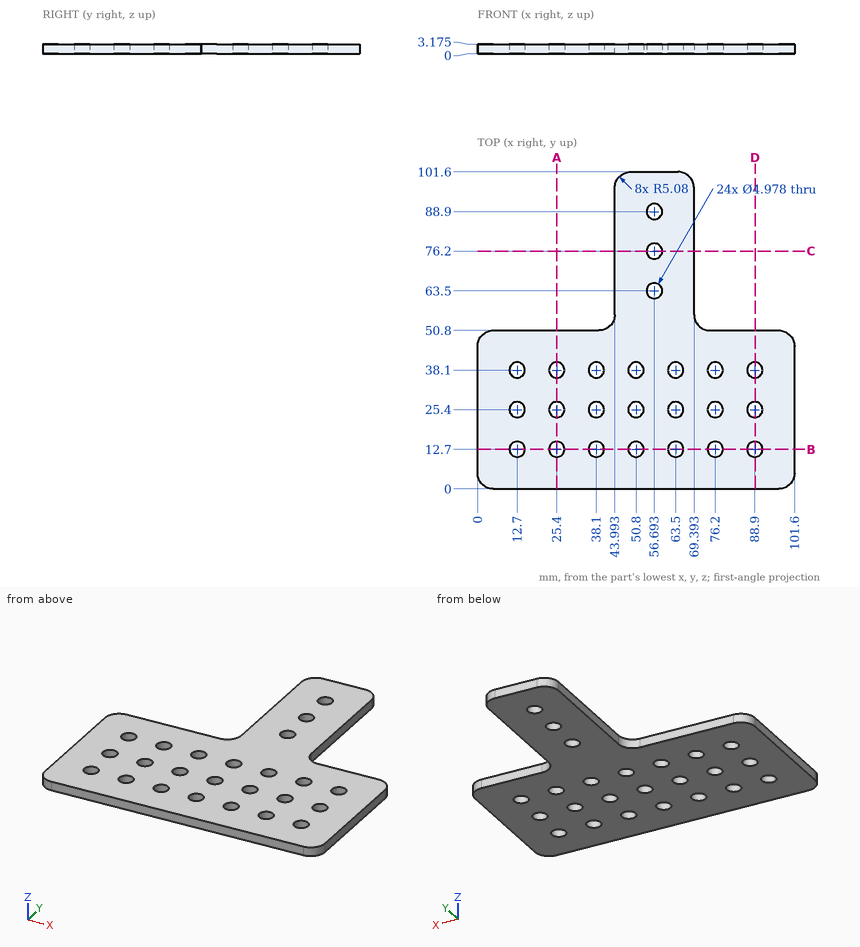
Here's the drawing with two shaded views (mm, measured from the low corner). I have some questions. Give positions to 0.01 mm unless a question says otherwise; leave off trailing zeros. Order: outer loops, then holes, each group sorted by start corner. A loop starts at its lowest first (then second) coordinate and runs counter-clockwise, first axis right, second up. Notation, with made-up numbers: (53, 13) - (65, 13) arc R28 cw to (65, 39) - close; hole circle Ø6 at (86.25, 12.25). An arc over 180 degrees is marked (long way). Write each question's results on one line, items separated by ' | '.
1) Suppose I cut it at A-A, the plane x = 25.4. Write out the boundary of the cut face in (y, z) (1 decimal), then the cut area to 3 significant figures.
Final values:
outline: (0, 0) - (10.2, 0) - (10.2, 3.2) - (0, 3.2) - close; (15.2, 0) - (22.9, 0) - (22.9, 3.2) - (15.2, 3.2) - close; (27.9, 0) - (35.6, 0) - (35.6, 3.2) - (27.9, 3.2) - close; (40.6, 0) - (50.8, 0) - (50.8, 3.2) - (40.6, 3.2) - close | area: 114 mm^2
2) Please list where these lines run through material, in increasing order: line 1 along Y through (x, z) = (63.5, 2.35); line 2 along Y through (x, z) = (74.5, 1.4); line 3 along X through (y, z) = (63.5, 1.65). Write a range as [from, to].
Final values:
line 1: y = [0, 10.21], [15.19, 22.91], [27.89, 35.61], [40.59, 101.6] | line 2: y = [0, 10.88], [14.52, 23.58], [27.22, 36.28], [39.92, 50.8] | line 3: x = [43.99, 54.2], [59.18, 69.39]
3) I'm going to push flat-ended pins straight in: pin 1 Ø3 at (x, y) = (54, 25.5) entering from -Z; pin 2 Ø1 at (x, z) = (19.5, 1.5) entering from +Y. Where does each tip first touch, or does it pass through?
Final values:
pin 1: stops at z = 0 | pin 2: stops at y = 50.8
4) Suppose I cut it at C-C, the plane y = 76.2. Write out the boundary of the cut face in (x, z) (1 decimal).
Final values:
outline: (44, 0) - (54.2, 0) - (54.2, 3.2) - (44, 3.2) - close; (59.2, 0) - (69.4, 0) - (69.4, 3.2) - (59.2, 3.2) - close
5) Suppose I cut it at B-B, the plane y = 12.7. Give the number of separate pieces and of enclosed holes in the cut face, then the cut area to 3 significant figures.
Final values:
separate pieces: 8 | enclosed holes: 0 | area: 212 mm^2
